```python
from build123d import *

# Parameters (mm, degrees)
ESQUISSE1_R      = 3
ESQUISSE1_R_2    = 1.25
ESQUISSE1_R_3    = 2.5
EXTRUSION1_DEPTH = 3


with BuildPart() as part:
    # Esquisse1 → Extrusion1 (new body)
    with BuildSketch(Plane(origin=(0, 0, 0), x_dir=(1, 0, 0), z_dir=(0, 1, 0))):
        with BuildLine():
            Line((-64.494367887, 52.858171056), (-99, 26))
            Line((-99, 26), (-104, 26))
            Line((-104, 26), (-104, 39))
            Line((-104, 39), (-124, 39))
            Line((-124, 39), (-124, 26))
            Line((-124, 26), (-131, 26))
            Line((-131, 26), (-131, 53))
            Line((-131, 53), (-101, 53))
            Line((-101, 53), (-101, 95))
            Line((-101, 95), (-83.5, 95))
            Line((-83.5, 95), (-83.5, 89))
            ThreePointArc((-83.5, 89), (-82.035533906, 85.464466094), (-78.5, 84))
            Line((-78.5, 84), (-28.5, 84))
            ThreePointArc((-28.5, 84), (-24.964466094, 85.464466094), (-23.5, 89))
            Line((-23.5, 89), (-23.5, 95))
            Line((-23.5, 95), (23.5, 95))
            Line((23.5, 95), (23.5, 89))
            ThreePointArc((23.5, 89), (24.964466094, 85.464466094), (28.5, 84))
            Line((28.5, 84), (78.5, 84))
            ThreePointArc((78.5, 84), (82.035533906, 85.464466094), (83.5, 89))
            Line((83.5, 89), (83.5, 95))
            Line((83.5, 95), (101, 95))
            Line((101, 95), (101, 53))
            Line((101, 53), (131, 53))
            Line((131, 53), (131, 26))
            Line((131, 26), (124, 26))
            Line((124, 26), (124, 39))
            Line((124, 39), (104, 39))
            Line((104, 39), (104, 26))
            Line((104, 26), (99, 26))
            Line((99, 26), (64.494367887, 52.858171056))
            ThreePointArc((64.494367887, 52.858171056), (0, 75), (-64.494367887, 52.858171056))
        make_face()
        with Locations((-91, 67)):
            Circle(ESQUISSE1_R, mode=Mode.SUBTRACT)
        with Locations((91, 67)):
            Circle(ESQUISSE1_R, mode=Mode.SUBTRACT)
        with Locations((-127.5, 45)):
            Circle(ESQUISSE1_R_2, mode=Mode.SUBTRACT)
        with Locations((-100.5, 45)):
            Circle(ESQUISSE1_R_2, mode=Mode.SUBTRACT)
        with Locations((-68.793992413, 58.382049127)):
            Circle(ESQUISSE1_R_3, mode=Mode.SUBTRACT)
        with Locations((68.793992413, 58.382049127)):
            Circle(ESQUISSE1_R_3, mode=Mode.SUBTRACT)
        with Locations((0, 85)):
            Circle(ESQUISSE1_R, mode=Mode.SUBTRACT)
        with Locations((-127.5, 29)):
            Circle(ESQUISSE1_R_2, mode=Mode.SUBTRACT)
        with Locations((-100.5, 29)):
            Circle(ESQUISSE1_R_2, mode=Mode.SUBTRACT)
        with Locations((100.5, 45)):
            Circle(ESQUISSE1_R_2, mode=Mode.SUBTRACT)
        with Locations((100.5, 29)):
            Circle(ESQUISSE1_R_2, mode=Mode.SUBTRACT)
        with Locations((127.5, 29)):
            Circle(ESQUISSE1_R_2, mode=Mode.SUBTRACT)
        with Locations((127.5, 45)):
            Circle(ESQUISSE1_R_2, mode=Mode.SUBTRACT)
    extrude(amount=EXTRUSION1_DEPTH)


solid = part.part
```
Input: part model. Units: mm. Frame: model coordinates. A direction names the side the tool comes from. Coordinates: 2 decimals unless noted, no trailing zeros. Write each loop counter-clockwise with the first axis right and the second up, starting at its lowest first coordinate (ties: lowest second). Pieces come first, ordered by that corner, then holes. Notation, with made-up numbers: (79, 67.25) -> (98, 67.25) arc R29 cw to (98, 87.25) -> close; hole circle Ø9 at (34.25, 36). An arc over 180 degrees is marked (long way). Answer as a JSON object with one key per item and string values.
1. Section A-A on x = 0. Return the cut outline in (y, z).
Result set:
{"outline": "(0, -95) -> (3, -95) -> (3, -88) -> (0, -88) -> close; (0, -82) -> (3, -82) -> (3, -75) -> (0, -75) -> close"}
2. Mould query, pull axis Z, two halves, no side actions, for faces 1 (the face through (2, 3, -76)), 2 (the face through (24.93, 1.48, -85.5)), 3 (the face through (-81.506, 1.479, -39.617)), 4 (the face through (-93.4, 1.5, -65.2)). Classes: released by +Z, released by -Z, zero draft, split by the parting line, or undercut.
Result set:
{"face 1": "zero draft", "face 2": "released by -Z", "face 3": "released by +Z", "face 4": "undercut"}
3. Material intervals for line 1 (Z direction, x = -127.5, y = 1.3); line 2 (Z direction, x = 100.5, y = 2.25); line 3 (X direction, y = 1.4, z = -35), sorted ascending. Write a range as from..to.
Result set:
{"line 1": "z = -53..-46.25, -43.75..-30.25, -27.75..-26", "line 2": "z = -95..-46.25, -43.75..-30.25, -27.75..-26", "line 3": "x = -131..-124, -104..-87.44, 87.44..104, 124..131"}
4. Access query for faces 5 (the face through (88.6, 1.5, -65.2)), 6 (the face through (81.99, 1.48, -39.24)), 7 (the face through (-25, 1.48, -85.43)). Directions: +Z, -Z, +X, -X, +Y, -Y. A direction counts if a zero-diameter tool reaches every point of the face in a straight line with its end or side. Return the directions, or none.
Result set:
{"face 5": "+Y, -Y", "face 6": "+Z, +Y, -Y", "face 7": "-Z, +Y, -Y"}
5. First-contact query: P1, Ø1.5, axis at x = -123.5, y = 1.5, coming from the -Z side; P2, Ø1.5, axis at x = 4.5, y = 2.5, coming from the +Z side; P3, Ø0.9, axis at x = 117, y = 1.5, coming from the +Z side. Flat tips, straight axial feed; report the tip coordinate or a pass-through.
Result set:
{"P1": "stops at z = -53", "P2": "stops at z = -74.87", "P3": "stops at z = -39"}
6. Section C-C on x = 91. Return the cut outline in (y, z), then the cut area to 3 significant figures.
Result set:
{"outline": "(0, -95) -> (3, -95) -> (3, -70) -> (0, -70) -> close; (0, -64) -> (3, -64) -> (3, -32.23) -> (0, -32.23) -> close", "area": "170 mm2"}
7. Section B-B on z = -36.5. Return the cut outline in (x, y), then the cut area to 3 significant figures.
Result set:
{"outline": "(-131, 0) -> (-124, 0) -> (-124, 3) -> (-131, 3) -> close; (-104, 0) -> (-85.51, 0) -> (-85.51, 3) -> (-104, 3) -> close; (85.51, 0) -> (104, 0) -> (104, 3) -> (85.51, 3) -> close; (124, 0) -> (131, 0) -> (131, 3) -> (124, 3) -> close", "area": "153 mm2"}
8. Section D-D on y = 2.5. Count the separate pieces of the cut face and the enclosed holes in it, then the cut area to 3 significant figures.
Result set:
{"separate pieces": "1", "enclosed holes": "13", "area": "7,240 mm2"}
